Input: part model. Units: mm. Frame: model coordinates. Coordinates: 2 decimals unless noted, no trailing zeros. Order: outer loops, then holes, each group sorted by start corner. A loop starts at its lowest first (then second) coordinate and runs counter-clockwise, first axis right, second up. Notation, with made-up numbers: (-32, 24) - (7, 24) arc R14 ccw to (7, 28) - close; hole circle Ø6 at (47, -38). An arc over 180 degrees is marked (long way). One line per question, with ' | ' between items.
from build123d import *

# Parameters (mm, degrees)
ESBO_O1_W                = 70
ESBO_O1_H                = 70
ESBO_O1_R                = 1.75
ESBO_O1_R_2              = 32.5
RESSALTO_EXTRUS_O1_DEPTH = 15.5


with BuildPart() as part:
    # Esboço1 → Ressalto-extrusão1 (new body)
    with BuildSketch(Plane.XY):
        Rectangle(ESBO_O1_W, ESBO_O1_H)
        with Locations((-31, -31)):
            Circle(ESBO_O1_R, mode=Mode.SUBTRACT)
        with Locations((31, -31)):
            Circle(ESBO_O1_R, mode=Mode.SUBTRACT)
        with Locations((31, 31)):
            Circle(ESBO_O1_R, mode=Mode.SUBTRACT)
        Circle(ESBO_O1_R_2, mode=Mode.SUBTRACT)
        with Locations((-31, 31)):
            Circle(ESBO_O1_R, mode=Mode.SUBTRACT)
    extrude(amount=RESSALTO_EXTRUS_O1_DEPTH)


solid = part.part
Item 1: Section A-A on y = -16.5. Return the cut outline in (x, z), and give its area (3 significant figures).
Data:
outline: (-35, 0) - (-28, 0) - (-28, 15.5) - (-35, 15.5) - close; (28, 0) - (35, 0) - (35, 15.5) - (28, 15.5) - close | area: 217 mm^2
Item 2: Contact query for a flat-ended pin moving along its axis: P1, Ø5.5, axis at x = 31, y = -31, coming from the -Z side. Output: stop coordinate, or through.
Data:
P1: z = 0
Item 3: Section D-D on y = -31. Return the cut outline in (x, z), and give its area (3 significant figures).
Data:
outline: (-35, 0) - (-32.75, 0) - (-32.75, 15.5) - (-35, 15.5) - close; (-29.25, 0) - (-9.76, 0) - (-9.76, 15.5) - (-29.25, 15.5) - close; (9.76, 0) - (29.25, 0) - (29.25, 15.5) - (9.76, 15.5) - close; (32.75, 0) - (35, 0) - (35, 15.5) - (32.75, 15.5) - close | area: 674 mm^2
Item 4: Draft query along Y for faces 1 (the face through (0, 35, 8)), 2 (the face through (-31, 11, 15.5)), 3 (the face through (-32.75, 31.08, 7.64)). Return one class per face: released by +Y, released by -Y, zero draft, split by the parting line, or undercut.
Data:
face 1: released by +Y | face 2: zero draft | face 3: undercut
Item 5: Section B-B on x = 26. Return the cut outline in (y, z).
Data:
outline: (-35, 0) - (-19.5, 0) - (-19.5, 15.5) - (-35, 15.5) - close; (19.5, 0) - (35, 0) - (35, 15.5) - (19.5, 15.5) - close
Item 6: Section C-C on z = 2. Return the cut outline in (x, y).
Data:
outline: (-35, -35) - (35, -35) - (35, 35) - (-35, 35) - close; hole circle Ø3.5 at (-31, -31); hole circle Ø3.5 at (-31, 31); hole circle Ø65 at (0, 0); hole circle Ø3.5 at (31, -31); hole circle Ø3.5 at (31, 31)
Item 7: Ray query, line 1 (Y direction, x = -1, z = 5); line 2 (Y direction, x = -28.5, z = 8.25); line 3 (X direction, y = -19.5, z = 8.75). Return the intervals inside material, ascending.
Data:
line 1: -35 to -32.48, 32.48 to 35 | line 2: -35 to -15.62, 15.62 to 35 | line 3: -35 to -26, 26 to 35
